Here's how the part is built. I have some questions about the finished solid (model axes, mm). A direction names the side the tool comes from. Round coordinates to 2 decimals unless told otherwise and drop trailing zeros. Write each loop counter-clockwise with the first axis right and the second up, starting at its lowest first coordinate (ties: lowest second). Pieces come first, ordered by that corner, then holes. Notation, with made-up numbers: (32.5, 68) - (45.5, 68) arc R18 ccw to (45.5, 72) - close; hole circle Ø8 at (-38.75, -33). An arc over 180 degrees is marked (long way). Use one line per item in the form item = value. Start each with the question number.
1. I want a section at B-B, the plane z = 84.5. List the corners of the cut face in (x, y) for me, plus the area to 3 significant figures.
2. We'd pull the mould along Z, two halves only. Please class faces 1 (the flat face through (1, 6, -127)), 2 (the flat face through (1, 12.7, -2)), 3 (the flat face through (30.695, 6.261, -63.781)): +Z half, -Z half, draft (parallel to the pull), parting line (faces both ways), or undercut.
3. Which directions (+Z, -Z, +X, -X, +Y, -Y) give clear straight access to the entire face, cutting with the end or side of a thin tool? Please do faces 4 (the cylindrical face through (-17.01, 6.26, -0.09)), 5 (the flat face through (-1, 6, 127)).
4. If I drill on line 1 along X through (y, z) = (7, -120.65); line 2 along Z through (x, y) = (-95.25, 9); line 3 along Z through (x, y) = (-59.69, 9), over which ranges is the centre line in solid material (lowest first)?
5. I want a section at C-C, the plane z = -47. List the corners of the cut face in (x, y) for me, plus the area to 3 significant figures.
6. I want a section at D-D, the plane y = 6. State how many separate pieces and enclosed holes the cut face has, plus the area to 3 significant figures.
7. I want a section at A-A, the plane x = 29. List the corners of the cut face in (y, z) for me (3 decimals), plus the area to 3 significant figures.
```python
from build123d import *

# Parameters (mm, degrees)
ORIGINAL_EXTRUSTION_DEPTH            = 12.7
HOLES_FOR_WHEELS_TO_MOUNT_DEPTH      = 164.134453749
HOLES_FOR_WHEELS_TO_MOUNT_DEPTH_BACK = 164.134453749
SKETCH2_R                            = 1.6


with BuildPart() as part:
    # Sketch1 → Original Extrustion (new body)
    # profile 1 of 4: a face of its own
    with BuildSketch(Plane(origin=(0, 0, 0), x_dir=(1, 0, 0), z_dir=(0, 1, 0))):
        Polygon((-101.6, 127), (0, 0), (101.6, 127), align=None)
        with BuildLine():
            ThreePointArc((-42.146144983, 111.125), (-53.592696084, 103.926496877), (-52.063178863, 90.491372896))
            Line((-52.063178863, 90.491372896), (-9.91703388, 37.808691667))
            ThreePointArc((-9.91703388, 37.808691667), (0, 33.042318771), (9.91703388, 37.808691667))
            Line((9.91703388, 37.808691667), (52.063178863, 90.491372896))
            ThreePointArc((52.063178863, 90.491372896), (53.592696084, 103.926496877), (42.146144983, 111.125))
            Line((42.146144983, 111.125), (-42.146144983, 111.125))
        make_face(mode=Mode.SUBTRACT)
    # profile 2 of 4: a face of its own
    with BuildSketch(Plane(origin=(0, 0, 0), x_dir=(1, 0, 0), z_dir=(0, 1, 0))):
        Polygon((0, 0), (-101.6, -127), (-101.6, 127), align=None)
        with BuildLine():
            Line((-90.4875, -67.080858304), (-90.4875, 67.080858304))
            ThreePointArc((-90.4875, 67.080858304), (-83.860454762, 76.428440433), (-72.846213574, 73.269087445))
            Line((-72.846213574, 73.269087445), (-19.181526931, 6.188229141))
            ThreePointArc((-19.181526931, 6.188229141), (-17.010813357, 0), (-19.181526931, -6.188229141))
            Line((-19.181526931, -6.188229141), (-72.846213574, -73.269087445))
            ThreePointArc((-72.846213574, -73.269087445), (-83.860454762, -76.428440433), (-90.4875, -67.080858304))
        make_face(mode=Mode.SUBTRACT)
    # profile 3 of 4: a face of its own
    with BuildSketch(Plane(origin=(0, 0, 0), x_dir=(1, 0, 0), z_dir=(0, 1, 0))):
        Polygon((-101.6, -127), (101.6, -127), (0, 0), align=None)
        with BuildLine():
            Line((-42.146144983, -111.125), (42.146144983, -111.125))
            ThreePointArc((42.146144983, -111.125), (53.592696084, -103.926496877), (52.063178863, -90.491372896))
            Line((52.063178863, -90.491372896), (9.91703388, -37.808691667))
            ThreePointArc((9.91703388, -37.808691667), (0, -33.042318771), (-9.91703388, -37.808691667))
            Line((-9.91703388, -37.808691667), (-52.063178863, -90.491372896))
            ThreePointArc((-52.063178863, -90.491372896), (-53.592696084, -103.926496877), (-42.146144983, -111.125))
        make_face(mode=Mode.SUBTRACT)
    # profile 4 of 4: a face of its own
    with BuildSketch(Plane(origin=(0, 0, 0), x_dir=(1, 0, 0), z_dir=(0, 1, 0))):
        Polygon((101.6, -127), (0, 0), (101.6, 127), align=None)
        with BuildLine():
            ThreePointArc((72.846213574, -73.269087445), (83.860454762, -76.428440433), (90.4875, -67.080858304))
            Line((90.4875, -67.080858304), (90.4875, 67.080858304))
            ThreePointArc((90.4875, 67.080858304), (83.860454762, 76.428440433), (72.846213574, 73.269087445))
            Line((72.846213574, 73.269087445), (19.181526931, 6.188229141))
            ThreePointArc((19.181526931, 6.188229141), (17.010813357, 0), (19.181526931, -6.188229141))
            Line((19.181526931, -6.188229141), (72.846213574, -73.269087445))
        make_face(mode=Mode.SUBTRACT)
    extrude(amount=ORIGINAL_EXTRUSTION_DEPTH)

    # Sketch2 → Holes for Wheels to mount (cut, two sides: drawn at the far end of the back side and taken through both)
    with BuildSketch(Plane(origin=(0, 12.7, 0), x_dir=(1, 0, 0), z_dir=(0, 1, 0)).offset(-HOLES_FOR_WHEELS_TO_MOUNT_DEPTH_BACK)):
        with Locations(Location((-95.25, 120.65, 0), (0, 0, 270))):
            Circle(SKETCH2_R)
        with Locations(Location((-59.69, 120.65, 0), (0, 0, 270))):
            Circle(SKETCH2_R)
        with Locations(Location((-95.25, 95.25, 0), (0, 0, 270))):
            Circle(SKETCH2_R)
        with Locations(Location((-59.69, 95.25, 0), (0, 0, 270))):
            Circle(SKETCH2_R)
        with Locations(Location((-95.25, -95.25, 0), (0, 0, 270))):
            Circle(SKETCH2_R)
        with Locations(Location((-59.69, -95.25, 0), (0, 0, 270))):
            Circle(SKETCH2_R)
        with Locations(Location((-95.25, -120.65, 0), (0, 0, 270))):
            Circle(SKETCH2_R)
        with Locations(Location((-59.69, -120.65, 0), (0, 0, 270))):
            Circle(SKETCH2_R)
        with Locations(Location((59.69, -95.25, 0), (0, 0, 270))):
            Circle(SKETCH2_R)
        with Locations(Location((95.25, -95.25, 0), (0, 0, 270))):
            Circle(SKETCH2_R)
        with Locations(Location((59.69, -120.65, 0), (0, 0, 270))):
            Circle(SKETCH2_R)
        with Locations(Location((95.25, -120.65, 0), (0, 0, 270))):
            Circle(SKETCH2_R)
        with Locations(Location((59.69, 120.65, 0), (0, 0, 270))):
            Circle(SKETCH2_R)
        with Locations(Location((59.69, 95.25, 0), (0, 0, 270))):
            Circle(SKETCH2_R)
        with Locations(Location((95.25, 95.25, 0), (0, 0, 270))):
            Circle(SKETCH2_R)
        with Locations(Location((95.25, 120.65, 0), (0, 0, 270))):
            Circle(SKETCH2_R)
    extrude(amount=HOLES_FOR_WHEELS_TO_MOUNT_DEPTH + HOLES_FOR_WHEELS_TO_MOUNT_DEPTH_BACK, mode=Mode.SUBTRACT)


solid = part.part
```
Model answer:
q1.outline = (-101.6, 0) - (-47.27, 0) - (-47.27, 12.7) - (-101.6, 12.7) - close; (47.27, 0) - (101.6, 0) - (101.6, 12.7) - (47.27, 12.7) - close
q1.area = 1,380 mm2
q2.face_1 = -Z half
q2.face_2 = draft
q2.face_3 = undercut
q3.face_4 = +Y, -Y
q3.face_5 = +Z, +X, -X, +Y, -Y
q4.line_1 = -101.6 to -96.85, -93.65 to -61.29, -58.09 to 58.09, 61.29 to 93.65, 96.85 to 101.6
q4.line_2 = -127 to -122.25, -119.05 to -96.85, -93.65 to 93.65, 96.85 to 119.05, 122.25 to 127
q4.line_3 = -127 to -122.25, -119.05 to -96.85, -93.65 to -56.82, 56.82 to 93.65, 96.85 to 119.05, 122.25 to 127
q5.outline = (-101.6, 0) - (-90.49, 0) - (-90.49, 12.7) - (-101.6, 12.7) - close; (-51.83, 0) - (-17.27, 0) - (-17.27, 12.7) - (-51.83, 12.7) - close; (17.27, 0) - (51.83, 0) - (51.83, 12.7) - (17.27, 12.7) - close; (90.49, 0) - (101.6, 0) - (101.6, 12.7) - (90.49, 12.7) - close
q5.area = 1,160 mm2
q6.separate_pieces = 1
q6.enclosed_holes = 20
q6.area = 26,600 mm2
q7.outline = (0, -127) - (12.7, -127) - (12.7, -111.125) - (0, -111.125) - close; (0, -61.662) - (12.7, -61.662) - (12.7, -18.461) - (0, -18.461) - close; (0, 18.461) - (12.7, 18.461) - (12.7, 61.662) - (0, 61.662) - close; (0, 111.125) - (12.7, 111.125) - (12.7, 127) - (0, 127) - close
q7.area = 1,500 mm2
